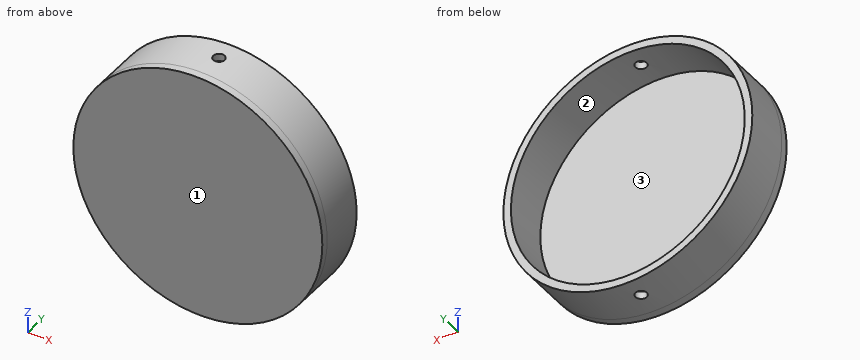
Autodesk Inventor part; units mm, degrees
ref_plane "Work Plane1" through (0, 0, 104.775) normal (0, 0, 1) x (1, 0, 0)
ref_plane "YZ Plane" through (0, 0, 0) normal (1, 0, 0) x (0, 1, 0)
ref_plane "XZ Plane" through (0, 0, 0) normal (0, 1, 0) x (-1, 0, 0)
sketch "Sketch1" plane through (0, 0, 0) normal (0, 1, 0) x (-1, 0, 0)
  circle A0 centre (0, 0) radius 104.775
  dimension "d0" = 209.55
extrude "Extrusion1" add sketch "Sketch1" against normal blind 6.35
sketch "Sketch2" plane through (0, 0, 0) normal (0, 1, 0) x (1, 0, 0)
  circle A0 centre (0, 0) radius 104.775
  circle A1 centre (0, 0) radius 104.775
  circle A2 centre (0, 0) radius 98.425
  dimension "d3" = 6.35
extrude "Extrusion2" add sketch "Sketch2" along normal blind 38.1
ref_plane "Work Plane1" through (0, 0, 104.775) normal (0, 0, 1) x (1, 0, 0)
sketch "Sketch3" plane through (0, 0, 104.775) normal (0, 0, 1) x (1, 0, 0)
  circle A0 centre (0, 20.9804) radius 4.7625
  line L0 (104.775, 38.1) -> (-104.775, 38.1)
  point P0 (0, 0)
  dimension "d6" = 9.525
  dimension "d7" = 17.1196
extrude "Extrusion3" cut sketch "Sketch3" against normal through all
properties part number "baseForBevelGearMount" material "Polycarbonate, Clear"
The model under review builds one solid part; all positions refer to its coordinate system, in mm. Face numbers are marked on the shaded views. Round coordinates to 2 decimals unless told otherwise and drop trailing zeros. Loops run counter-clockwise (first coordinate to the right, second up) from the corner with the lowest first, then second, coordinate; pieces in that order, holes last. Notation, with made-up numbers: M -40,15 L -32,15 A10 ccw -32,27 Z; hole C 31,73.25 d1. An arc over 180 degrees is marked long. Write item = value, one per line.
Item 1: Insertion check: P1, Ø2, axis at x = -20.5, y = 18, coming from the +Z side; P2, Ø8, axis at x = -60.5, y = 16, coming from the +Z side; P3, Ø3, axis at y = 8, z = 50, coming from the -X side; P4, Ø15, axis at x = 0, y = 20.98, coming from the +Z side (3 decimals). Each pin has a flat end and moves straight along its axis. Give the tip position at first contact, or say it passes through.
Return value:
P1 = 102.94
P2 = 88.24
P3 = -92.87
P4 = 104.775
Item 2: Take a section at D-D on x = 37.5. Write out the cut boundary in (y, z), then the cut area to 3 significant figures.
Return value:
outline = M -6.35,-97.83 L 38.1,-97.83 L 38.1,-91 L 0,-91 L 0,91 L 38.1,91 L 38.1,97.83 L -6.35,97.83 Z
area = 1,760 mm2
Item 3: The part is to be moulded in two halves that separate along Z. For the marked faces 1, 2 and 3, say which applies: released by +Z, released by -Z, zero draft, split by the parting line, or undercut.
Return value:
face_1 = zero draft
face_2 = undercut
face_3 = undercut
Item 4: For line 1 (Y direction, x = 0, z = 103); line 2 (X direction, y = 30.5, z = 0) (3 decimals); line 3 (Z direction, x = -70, y = 11.5), list the stretches that pass through material, from the lowest coordinate up. Write a range as [from, to].
Return value:
line_1 = [-6.35, 16.22], [25.74, 38.1]
line_2 = [-104.775, -98.425], [98.425, 104.775]
line_3 = [-77.96, -69.19], [69.19, 77.96]
Item 5: Take a section at A-A on x = 0. Write out the cut boundary in (y, z) (3 decimals), then the cut area to 3 significant figures.
Return value:
outline = M -6.35,-104.775 L 16.218,-104.775 L 16.218,-98.425 L 0,-98.425 L 0,98.425 L 16.218,98.425 L 16.218,104.775 L -6.35,104.775 Z; M 25.743,-104.775 L 38.1,-104.775 L 38.1,-98.425 L 25.743,-98.425 Z; M 25.743,98.425 L 38.1,98.425 L 38.1,104.775 L 25.743,104.775 Z
area = 1,690 mm2
Item 6: Take a section at C-C on y = 31. Write out the cut boundary in (x, z) (3 decimals).
Return value:
outline = C 0,0 d209.55; hole C 0,0 d196.85
Item 7: Take a section at B-B on z = 0. Write out the cut boundary in (x, y) (3 decimals), then the cut area to 3 significant figures.
Return value:
outline = M -104.775,-6.35 L 104.775,-6.35 L 104.775,38.1 L 98.425,38.1 L 98.425,0 L -98.425,0 L -98.425,38.1 L -104.775,38.1 Z
area = 1,810 mm2
